```python
from build123d import *

# Parameters (mm, degrees)
SKETCH1_R           = 65
BOSS_EXTRUDE1_DEPTH = 5
SKETCH2_R           = 57
CUT_EXTRUDE1_DEPTH  = 5
SKETCH3_R           = 4.5
BOSS_EXTRUDE2_DEPTH = 28
BOSS_EXTRUDE3_DEPTH = 19
CUT_EXTRUDE2_DEPTH  = 10


with BuildPart() as part:
    # Sketch1 → Boss-Extrude1 (new body)
    with BuildSketch(Plane(origin=(0, 0, 0), x_dir=(0, 0, -1), z_dir=(1, 0, 0))):
        Circle(SKETCH1_R)
    extrude(amount=BOSS_EXTRUDE1_DEPTH)

    # Sketch2 → Cut-Extrude1 (cut)
    with BuildSketch(Plane(origin=(5, 0, 0), x_dir=(0, 0, -1), z_dir=(1, 0, 0))):
        with Locations((0, 65)):
            Circle(SKETCH2_R)
    extrude(amount=-CUT_EXTRUDE1_DEPTH, mode=Mode.SUBTRACT)

    # Sketch3 → Boss-Extrude2 (add)
    with BuildSketch(Plane(origin=(5, 0, 0), x_dir=(0, 0, -1), z_dir=(1, 0, 0))):
        Circle(SKETCH3_R)
    extrude(amount=BOSS_EXTRUDE2_DEPTH)

    # Sketch4 → Boss-Extrude3 (add)
    with BuildSketch(Plane(origin=(5, 0, 0), x_dir=(0, 0, -1), z_dir=(1, 0, 0))):
        with BuildLine():
            Line((-38.528819584, -41.954177593), (-39.717618419, -41.296537903))
            add(Edge.make_bspline(
                [(-39.717618419, -41.296537903), (-19.85880921, 8), (0, 8)],
                knots=[0, 0, 0, 1, 1, 1], degree=2))
            Line((0, 8), (-1.834255985, 6.832495808))
            add(Edge.make_bspline(
                [(-38.528819584, -41.954177593), (-19.49735867, 4.777398316), (-1.834255985, 6.832495808)],
                knots=[0, 0, 0, 1, 1, 1], degree=2))
        make_face()
    extrude(amount=BOSS_EXTRUDE3_DEPTH)

    # Sketch5 → Cut-Extrude2 (cut)
    with BuildSketch(Plane.ZY):
        with BuildLine():
            add(Edge.make_bspline(
                [(-59.611313459, 41.161832135), (-62.271021167, 28.272133344), (0.725304908, -12.45080433), (121.126777355, 64.589791019), (-54.876290799, 64.109096486), (-59.611313459, 41.161832135)],
                knots=[0, 0, 0, 0, 0.262262558, 0.533099388, 1, 1, 1, 1], degree=3))
        make_face()
    extrude(amount=-CUT_EXTRUDE2_DEPTH, mode=Mode.SUBTRACT)


solid = part.part
```
Design review of the part built by this model. Coordinates are the model's own, in mm. Coordinates: 2 decimals unless noted, no trailing zeros. Order: outer loops, then holes, each group sorted by start corner. A loop starts at its lowest first (then second) coordinate and runs counter-clockwise, first axis right, second up.
1) Take a section at A-A, the plane x = 26. Give the boundary of the cut face in (y, z).
2) Wall thickness on line 1 along X through (y, z) = (-4, 24.5); line 2 along Y through (x, z) = (12, -0.5); line 3 along Y through (x, z) = (3.5, 15.5): over which ranges is each line inside the solid? List them lowest first.
3) Clearance check with flat-ended pins moving along their axes: pin 1 (2 mm diameter, centred on x = 9, y = -19.5, fed in from -Z); pin 2 (5 mm diameter, centred on y = -40.5, z = 7, fed in from -X); pin 3 (3 mm diameter, centred on x = 13, y = -38, fed in from -Z); pin 4 (4 mm diameter, centred on x = 4, z = 48, fed in from -Y). State where each tip first meets the part, or that it passes through.
4) Mouldability with a two-part tool opening along Y and no side actions: class faces 1 (the flat face through (24, -15, 26)), 2 (the cylindrical face through (18.8, 4.46, 0.59)), 3 (the cylindrical face through (2.535, 8.027, -1.756)), 4 (the cylindrical face through (2.46, -64.99, 1.06)) as +Y half, -Y half, draft (parallel to the pull), parting line (faces both ways), or undercut.
5) Take a section at B-B, the plane y = -52.5. Give the boundary of the cut face in (x, z).
Returned:
1. outline: circle Ø9 at (0, 0)
2. line 1: x = 0 to 5
2. line 2: y = -4.47 to 4.47
2. line 3: y = -63.12 to 9.41
3. pin 1: stops at z = 27.55
3. pin 2: stops at x = 0
3. pin 3: stops at z = 36.25
3. pin 4: stops at y = -45.92
4. face 1: draft
4. face 2: undercut
4. face 3: +Y half
4. face 4: parting line
5. outline: (0, -38.32) - (5, -38.32) - (5, 38.32) - (0, 38.32) - close
